Check sheet for the drawn part. Datum: minimum x, y, z corner. Units: mm. A direction names the side the tool comes from. Give positions to 0.01 mm unless a question says otherwise; leave off trailing zeros. Loops run counter-clockwise (first coordinate to the right, second up) from the corner with the lowest first, then second, coordinate; pieces in that order, holes last. Notation, with made-up numbers: (2.25, 21.25) -> (52.25, 21.25) arc R24 cw to (52.25, 59.25) -> close; hole circle Ø9 at (53.25, 36). An arc over 180 degrees is marked (long way). One line per question, with ' | ' between items.
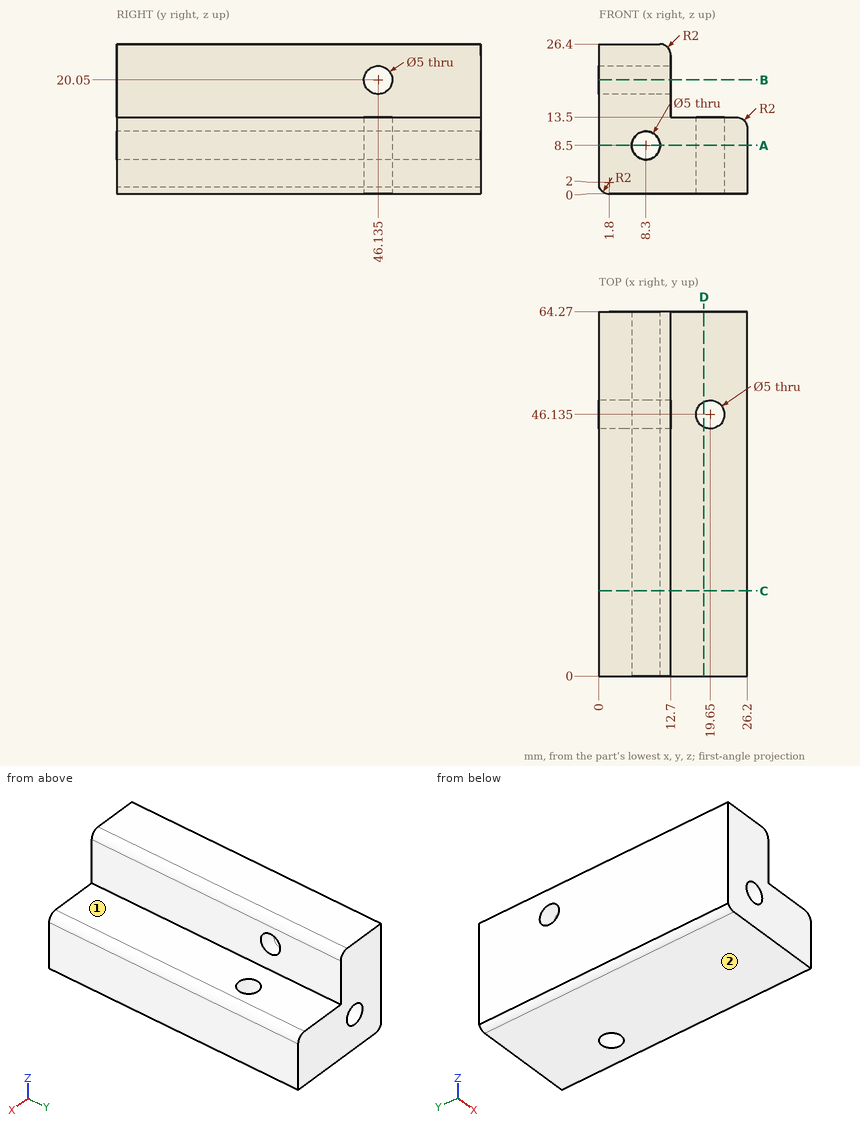
Item 1: Sectioned sample at A-A (z = 8.5). Record the cut outline in (x, y) (3 decimals), plus the area to 3 significant figures.
Result:
outline: (0, 0) -> (5.8, 0) -> (5.8, 64.27) -> (0, 64.27) -> close; (10.8, 0) -> (26.2, 0) -> (26.2, 64.27) -> (10.8, 64.27) -> close; hole circle Ø5 at (19.65, 46.135) | area: 1,340 mm2
Item 2: Depth check by flat-ended pin: pin 1 Ø3 at (y, z) = (46.135, 20.05) entering from -X (3 decimals); pin 2 Ø6 at (x, z) = (8.3, 8.5) entering from +Y; pin 3 Ø3.5 at (y, z) = (27.5, 18.5) entering from +X; pin 4 Ø5.5 at (x, y) = (17, 25.5) entering from +Z. Enter the tip coordinate at first touch or a pass-through.
Result:
pin 1: through | pin 2: y = 64.27 | pin 3: x = 12.7 | pin 4: z = 13.5
Item 3: Sectioned sample at B-B (z = 20.05). Record the cut outline in (x, y) (3 decimals).
Result:
outline: (0, 0) -> (12.7, 0) -> (12.7, 43.635) -> (0, 43.635) -> close; (0, 48.635) -> (12.7, 48.635) -> (12.7, 64.27) -> (0, 64.27) -> close
Item 4: Set-up check for the marked faces 1 and 2: record each of +Z, -Z, +X, -X, +Y, -Y from which the full face is reachable in a straight line by a thin tool's end or side.
Result:
face 1: +Z, +X, +Y, -Y | face 2: -Z, +X, -X, +Y, -Y
Item 5: Sectioned sample at C-C (y = 15). Record the cut outline in (x, z).
Result:
outline: (0, 1.13) arc R2 ccw to (1.8, 0) -> (26.2, 0) -> (26.2, 11.5) arc R2 ccw to (24.2, 13.5) -> (12.7, 13.5) -> (12.7, 24.4) arc R2 ccw to (10.7, 26.4) -> (0, 26.4) -> close; hole circle Ø5 at (8.3, 8.5)
Item 6: Sectioned sample at D-D (x = 18.5). Record the cut outline in (y, z), plus the area to 3 significant figures.
Result:
outline: (0, 0) -> (43.92, 0) -> (43.92, 13.5) -> (0, 13.5) -> close; (48.35, 0) -> (64.27, 0) -> (64.27, 13.5) -> (48.35, 13.5) -> close | area: 808 mm2
Item 7: Scan lines: probe 1 along Z at (x, y) = (8.3, 49.5); probe 2 along Y at (x, z) = (10.2, 20.05) (3 decimals); probe 3 along Z at (x, y) = (15, 30.5). Record each from-to range of solid material in increasing order.
Result:
probe 1: 0 to 6, 11 to 26.4 | probe 2: 0 to 43.635, 48.635 to 64.27 | probe 3: 0 to 13.5
